Autodesk Inventor part; units mm, degrees
ref_plane "YZ Plane" through (0, 0, 0) normal (1, 0, 0) x (0, 1, 0)
ref_plane "XZ Plane" through (0, 0, 0) normal (0, 1, 0) x (-1, 0, 0)
ref_plane "XY Plane" through (0, 0, 0) normal (0, 0, 1) x (1, 0, 0)
sketch "Sketch1" plane through (0, 0, 0) normal (0, 1, 0) x (-1, 0, 0)
  line L0 (216, 0) -> (266.75, 0)
  line L1 (266.75, 0) -> (266.75, 2)
  line L2 (266.75, 2) -> (355, 2)
  line L3 (355, 2) -> (355, 60.5)
  line L4 (355, 60.5) -> (216, 60.5)
  line L5 (216, 60.5) -> (216, 0)
  line L6 (0, 0) -> (0, 60.5)
  line L7 (0, 60.5) -> (216, 60.5) construction
  line L8 (0, 0) -> (216, 0) construction
  line L9 (-457, 457) -> (-396.5, 457) construction
  line L10 (-396.5, 457) -> (-396.5, 673) construction
  line L11 (-396.5, 673) -> (-457, 673)
  line L12 (-457, 673) -> (-457, 457) construction
  line L13 (-396.5, 673) -> (-396.5, 812)
  line L14 (-396.5, 812) -> (-455, 812)
  line L15 (-455, 812) -> (-455, 723.75)
  line L16 (-455, 723.75) -> (-457, 723.75)
  line L17 (-457, 723.75) -> (-457, 673)
  dimension "d0" = 432
  dimension "d1" = 710
  dimension "d2" = 533.5
  dimension "d3" = 2
  dimension "d4" = 60.5
  dimension "d6" = 2
  dimension "d7" = 60.5
  dimension "d8" = 432
  dimension "d9" = 533.5
  dimension "d10" = 710
  dimension "d11" = 457
  dimension "d12" = 457
revolve "Revolution1" add sketch "Sketch1" angle 360 about axis through (0, 0, 0) along (0, 0, 1) contours L5 L4 L3 L2 L1 L0
revolve "Revolution2" add sketch "Sketch1" angle 360 about axis through (457, 0, 457) along (-1, 0, 0) contours L11 L17 L16 L15 L14 L13
sketch "Sketch2" plane through (0, 0, 0) normal (0, 1, 0) x (-1, 0, 0)
  line L0 (-396.5, 673) -> (-396.5, 812)
  line L1 (355, 60.5) -> (216, 60.5)
  line L2 (0, 0) -> (0, 60.5)
  line L3 (-457, 457) -> (-396.5, 457)
  arc A0 (0, 60.5) -> (-396.5, 457) centre (-396.5, 60.5) ccw
sketch "Sketch3" plane through (0, 0, 60.5) normal (0, 0, 1) x (1, 0, 0)
  circle A0 centre (0, 0) radius 216
  circle A1 centre (0, 0) radius 216
  circle A2 centre (0, 0) radius 235
  dimension "d14" = 470
sweep "Sweep1" add profiles "Sketch3" path "Sketch2" path curves L2 A0 L3
sketch "Sketch6" plane through (0, 0, 2) normal (0, 0, -1) x (-1, 0, 0)
  circle A0 centre (0, 0) radius 355
  circle A1 centre (-41.0179, -311.5615) radius 17.75
  circle A2 centre (0, 0) radius 314.25 construction
  line L0 (-41.0179, -311.5615) -> (0, 0) construction
  line L1 (0, 0) -> (0, -314.25) construction
  dimension "d20" = 7.5
  dimension "d21" = 35.5
  dimension "d22" = 628.5
extrude "Extrusion1" cut sketch "Sketch6" against normal up to surface (58.5 mm away) contours A1
pattern_circular "Circular Pattern1" count 24 over 360 about axis through (0, 0, 31.25) along (0, 0, -1) of "Extrusion1"
sketch "Sketch7" plane through (455, 0, 457) normal (1, 0, 0) x (0, 0, -1)
  circle A0 centre (0, 0) radius 266.75
  circle A1 centre (-41.0179, -311.5615) radius 17.75
  circle A2 centre (0, 0) radius 314.25 construction
  line L0 (-41.0179, -311.5615) -> (0, 0) construction
  line L1 (0, 0) -> (0, -314.25) construction
  dimension "d25" = 7.5
  dimension "d26" = 35.5
  dimension "d27" = 628.5
extrude "Extrusion2" cut sketch "Sketch7" against normal up to surface (58.5 mm away) contours A1
pattern_circular "Circular Pattern2" count 24 over 360 about axis through (425.75, 0, 457) along (-1, 0, 0) of "Extrusion2"
equation "\"d0\" = d"
equation "\"d1\" = D1"
equation "\"d2\" = D2"
equation "\"d4\" = C1"
equation "\"d7\" = C1"
equation "\"d8\" = d"
equation "\"d9\" = D2"
equation "\"d10\" = D1"
equation "\"d11\" = AA"
equation "\"d12\" = AA"
equation "\"d14\" = d + 2 * t"
equation "\"d21\" = L"
equation "\"d22\" = K1"
equation "\"d26\" = L"
equation "\"d27\" = K1"
equation "\"D1\" = 710"
equation "\"C1\" = 60.5"
equation "\"t\" = 19"
equation "\"d\" = 432"
equation "\"AA\" = 457"
equation "\"D2\" = 533.5"
equation "\"K1\" = 628.5"
equation "\"L\" = 35.5"
properties part number "GB/T 17185 450-PN50 \"F90E(S) RF\"" material "Steel"
Source: CAD feature listing. Evaluate the final solid. Frame: model axes, mm. A direction names the side the tool comes from. Give positions to 0.01 mm unless a question says otherwise; leave off trailing zeros. Write each loop counter-clockwise with the first axis right and the second up, starting at its lowest first coordinate (ties: lowest second). Pieces come first, ordered by that corner, then holes. Notation, with made-up numbers: (1.25, 72) - (24.25, 72) arc R24 ccw to (24.25, 106) - close; hole circle Ø11 at (53.5, 87.25). An arc over 180 degrees is marked (long way). One line per item, written item: value. Start each with the question number.
Q1. Draft query along X for faces 4 (the face through (426.16, -199.505, 690.57)), 5 (the face through (-188.98, -266.91, 30.84)). Return one class per face: +X half, -X half, draft (parallel to the pull), parting line (faces both ways), or undercut.
Q2. Set-up query: faces 1 (the face through (456.014, -80.124, 711.432)), 2 (the face through (46.825, -210.864, 29.826)), 3 (the face through (-180.503, 263.397, 30.84)). Return all of +Z, -Z, +X, -X, +Y, -Y with unobstructed straight access to the full face (end or side cutting, diameter ignored); none if empty.
Q3. Material intervals for probe 1 along Y at (x, z) = (401, 208.5); probe 2 along X at (y, z) = (-68.5, 129); probe 3 along Z at (x, y) = (268, -121.5), sorted ascending. Write a range as from..to.
Q4. First-contact query: pin 1 Ø6 at (x, y) = (80.5, 113.5) entering from -Z; pin 2 Ø10 at (x, y) = (-134, 94) entering from +Z; pin 3 Ø12 at (y, z) = (151.5, 528) entering from -X. Flat tips, straight axial feed; report the tip coordinate or a pass-through.
Q5. Section query A-A, the plane y = 0. Return the cut outline in (x, z), then the cut area to 3 significant figures.
Answer:
1. face 4: draft
1. face 5: undercut
2. face 1: +X
2. face 2: -Z
2. face 3: +Z, -Z
3. probe 1: y = -253.52..-209.03, -173.57..173.57, 209.03..253.52
3. probe 2: x = -221.01..-200.94, 217.51..239.05, 396.5..455
3. probe 3: z = 2..60.5, 207.63..236.49, 621.05..644.18
4. pin 1: stops at z = 544.21
4. pin 2: stops at z = 374.93
4. pin 3: stops at x = 48.11
5. outline: (-355, 2) - (-266.75, 2) - (-266.75, 0) - (-216, 0) - (-216, 60.5) arc R612.5 cw to (396.5, 673) - (457, 673) - (457, 723.75) - (455, 723.75) - (455, 812) - (396.5, 812) - (396.5, 692) arc R631.5 ccw to (-235, 60.5) - (-355, 60.5) - close; (216, 0) - (266.75, 0) - (266.75, 2) - (355, 2) - (355, 60.5) - (235, 60.5) arc R161.5 cw to (396.5, 222) - (396.5, 102) - (455, 102) - (455, 190.25) - (457, 190.25) - (457, 241) - (396.5, 241) arc R180.5 ccw to (216, 60.5) - close
5. area: 56,600 mm2
